from build123d import *

# Parameters (mm, degrees)
F0_R     = 3.175
F1_DEPTH = 3.175


with BuildPart() as f1:
    # F0 (on Top) → F1 (new body)
    with BuildSketch(Plane.XY):
        with BuildLine():
            ThreePointArc((-4.6690304578, 36.0608687482), (-4.926356626, 42.1933740702), (-10.2528819721, 45.2432865312))
            ThreePointArc((-10.2528819721, 45.2432865312), (-13.6512609491, 44.3196488769), (-16.034861924, 41.7272498758))
            ThreePointArc((-16.034861924, 41.7272498758), (-24.6382163154, 8.2639214044), (-18.7919287035, -25.7894628669))
            Line((-18.7919287035, -25.7894628669), (-12.3928580021, 2.7761611158))
            ThreePointArc((-12.3928580021, 2.7761611158), (-12.2172281013, 3.4683335365), (-12.0029711474, 4.1495401716))
            ThreePointArc((-12.0029711474, 4.1495401716), (-10.2322760444, 20.5410111397), (-4.6690304578, 36.0608687482))
        make_face()
        with BuildLine():
            ThreePointArc((-7.1769461909, 38.894059312), (-12.6144546933, 36.6665763656), (-10.3024140815, 42.0686729216))
            ThreePointArc((-10.3024140815, 42.0686729216), (-8.0894376884, 41.1215422584), (-7.1769461909, 38.894059312))
        make_face(mode=Mode.SUBTRACT)
        with BuildLine():
            ThreePointArc((-18.7919287035, -25.7894628669), (-17.199620286, -29.5004662895), (-15.4277360093, -33.1291600779))
            ThreePointArc((-15.4277360093, -33.1291600779), (-10.0074027219, -36.507133329), (-4.3842812821, -39.5355357964))
            ThreePointArc((-4.3842812821, -39.5355357964), (-1.4791469298, -35.6407535094), (-2.1779859288, -30.8323485013))
            ThreePointArc((-2.1779859288, -30.8323485013), (-9.4049707621, -13.9914505961), (-12.0029711474, 4.1495401716))
            ThreePointArc((-12.0029711474, 4.1495401716), (-12.2172281013, 3.4683335365), (-12.3928580021, 2.7761611158))
            Line((-12.3928580021, 2.7761611158), (-18.7919287035, -25.7894628669))
        make_face()
        with Locations((-7.6344430684, -34.0803595057)):
            Circle(F0_R, mode=Mode.SUBTRACT)
        with BuildLine():
            ThreePointArc((-4.3842812821, -39.5355357964), (-10.0074027219, -36.507133329), (-15.4277360093, -33.1291600779))
            ThreePointArc((-15.4277360093, -33.1291600779), (-14.2898816566, -35.2457737279), (-13.0909002079, -37.32837051))
            ThreePointArc((-13.0909002079, -37.32837051), (-9.1948370721, -40.2356556442), (-4.3842812821, -39.5355357964))
        make_face()
    extrude(amount=F1_DEPTH)


solid = f1.part
Work out the finished part from the listing and answer in its coordinate system (mm). Give positions to 0.01 mm unless a question says otherwise; leave off trailing zeros. Loops run counter-clockwise (first coordinate to the right, second up) from the corner with the lowest first, then second, coordinate; pieces in that order, holes last. Notation, with made-up numbers: (39, 89) - (57, 89) arc R16 ccw to (57, 115) - close; hole circle Ø11 at (-5.75, 33). An arc over 180 degrees is marked (long way). Answer in a Markdown table with one row per item. Add a question column.
Q1. The part is cut by section A-A (z = 1.55). Determine the outline of the cut face in (x, y) (3 decimals), and give its area (3 significant figures).
Q2. The part is cut by section B-B (y = -30). Determine the outline of the cut face in (x, z) (3 decimals).
Q3. The part is cut by section C-C (x = -20.5). Determine the outline of the cut face in (y, z) (1 decimal).
Q4. Consider line 1 along Y through (x, z) = (-5.25, 2); line 2 along X through (y, z) = (6, 0.25); line 3 along X through (y, z) = (-34, 0.7). Determine where each line is inside the solid, lowest interval first.
Solution:
| question | item | result |
|---|---|---|
| 1 | outline | (-16.035, 41.727) arc R82.55 ccw to (-13.091, -37.328) arc R6.35 ccw to (-2.178, -30.832) arc R69.85 cw to (-4.669, 36.061) arc R6.35 ccw to start; hole circle Ø6.35 at (-10.352, 38.894); hole circle Ø6.35 at (-7.634, -34.08) |
| 1 | area | 1,030 mm² |
| 2 | outline | (-16.969, 0) - (-2.666, 0) - (-2.666, 3.175) - (-16.969, 3.175) - close |
| 3 | outline | (-21.1, 0) - (30.9, 0) - (30.9, 3.2) - (-21.1, 3.2) - close |
| 4 | line 1 | y = -39.97 to -36.18, -31.98 to -25.08, 34.87 to 42.67 |
| 4 | line 2 | x = -24.7 to -12 |
| 4 | line 3 | x = -14.97 to -10.81, -4.46 to -1.28 |
